Can you work these out from the model? Positions are in its coordinate system, mm. Give positions to 0.01 mm unless a question says otherwise; leave off trailing zeros. Loops run counter-clockwise (first coordinate to the right, second up) from the corner with the lowest first, then second, coordinate; pieces in that order, holes last. Notation, with made-up numbers: M 11.25,-9.75 L 25.25,-9.75 A15 ccw 25.25,10.25 Z; hole C 33,89.5 d9. An arc over 180 degrees is marked long. Answer as a JSON object with one key per item and string values.
```python
from build123d import *

# Parameters (mm, degrees)
SKETCH1_W          = 350
SKETCH1_H          = 6
TAPPED_HOLE1_D     = 3.3
TAPPED_HOLE1_DEPTH = 11.5
TAPPED_HOLE1_TIP   = 0.991420021
TAPPED_HOLE2_D     = 3.3
TAPPED_HOLE2_DEPTH = 11.5
TAPPED_HOLE2_TIP   = 0.991420021
CHAMFER1_SIZE      = 0.5


with BuildPart() as part:
    # Sketch1 → Revolve1 (revolve)
    with BuildSketch(Plane.XY, mode=Mode.PRIVATE) as revolve1_sk:
        with Locations((175, 3)):
            Rectangle(SKETCH1_W, SKETCH1_H)
    revolve(revolve1_sk.sketch.rotate(Axis((0, 0, 0), (1, 0, 0)), 90), axis=Axis((0, 0, 0), (1, 0, 0)))

    # Tapped Hole1
    with Locations(Plane.ZY):
        with Locations((0, 0)):
            Hole(TAPPED_HOLE1_D / 2, depth=TAPPED_HOLE1_DEPTH)
            with Locations((0, 0, -(TAPPED_HOLE1_DEPTH + TAPPED_HOLE1_TIP / 2))):  # 118° drill point
                Cone(0, TAPPED_HOLE1_D / 2, TAPPED_HOLE1_TIP, mode=Mode.SUBTRACT)

    # Tapped Hole2
    with Locations(Plane(origin=(350, 0, 0), x_dir=(0, 0, -1), z_dir=(1, 0, 0))):
        with Locations((0, 0)):
            Hole(TAPPED_HOLE2_D / 2, depth=TAPPED_HOLE2_DEPTH)
            with Locations((0, 0, -(TAPPED_HOLE2_DEPTH + TAPPED_HOLE2_TIP / 2))):  # 118° drill point
                Cone(0, TAPPED_HOLE2_D / 2, TAPPED_HOLE2_TIP, mode=Mode.SUBTRACT)

    # Chamfer1
    chamfer1_edges = [part.edges().sort_by_distance(p)[0] for p in [
        (350, 0, -6),
        (0, 0, -6),
    ]]
    chamfer(chamfer1_edges, length=CHAMFER1_SIZE)


solid = part.part
```
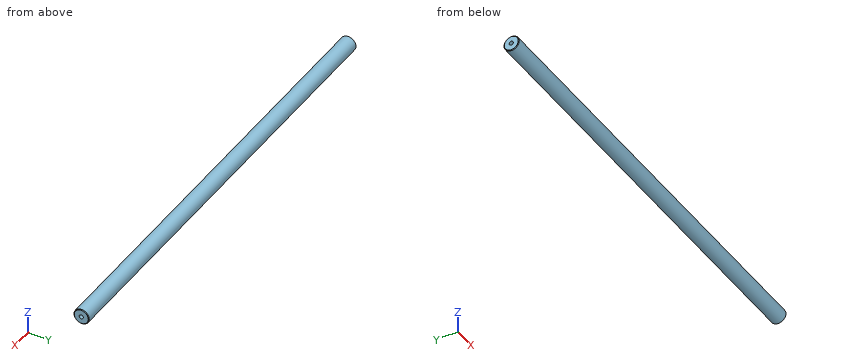
1) Will these pins go through, and if not, where does the flat tip stop? pin 1 Ø5 at (x, z) = (94.5, -4.5) entering from -Y; pin 2 Ø1 at (x, y) = (215.5, 2.5) entering from +Z.
Answer list:
{"pin 1": "y = -5.66", "pin 2": "z = 5.66"}
2) Suppose I cut it at A-A, the plane x = 172.5. Write out the boundary of the cut face in (y, z).
Answer list:
{"outline": "C 0,0 d12"}
3) Please list where these lines run through material, in increasing order: line 1 along Y through (x, z) = (2.5, 0); line 2 along Y through (x, z) = (77.5, -2.5); line 3 along X through (y, z) = (-3.5, 4.25). Write a range as from..to.
Answer list:
{"line 1": "-6..-1.65, 1.65..6", "line 2": "-5.45..5.45", "line 3": "0.01..349.99"}
